Geometry check sheet. Reference: the model listing, model coordinates, mm. A direction names the side the tool comes from. Coordinates: 2 decimals unless noted, no trailing zeros. Write each loop counter-clockwise with the first axis right and the second up, starting at its lowest first coordinate (ties: lowest second). Pieces come first, ordered by that corner, then holes. Notation, with made-up numbers: M -19.75,67.5 L 36.25,67.5 A16 ccw 36.25,88.5 Z; hole C 71.25,-27 d3. An arc over 180 degrees is marked long. Write each question's results on one line, items separated by ' | '.
```python
from build123d import *

# Parameters (mm, degrees)
BOSS_EXTRUDE1_DEPTH = 38.1
SKETCH2_W           = 38.1
SKETCH2_H           = 22.225
BOSS_EXTRUDE2_DEPTH = 25.4
CUT_EXTRUDE1_DEPTH  = 25.4


with BuildPart() as part:
    # Sketch1 → Boss-Extrude1 (new body, symmetric)
    with BuildSketch(Plane(origin=(0, 0, 0), x_dir=(0, 0, -1), z_dir=(1, 0, 0))):
        Polygon((-10.0584, -30.4038), (8.9916, -30.4038), (8.9916, -52.6288), (34.3916, -52.6288), (34.3916, 14.0462), (8.9916, 14.0462), (8.9916, -8.1788), (-10.0584, -8.1788), align=None)
    extrude(amount=BOSS_EXTRUDE1_DEPTH, both=True)

    # Sketch2 → Boss-Extrude2 (add)
    with BuildSketch(Plane.XY.offset(10.0584)):
        with Locations((0, -19.2913)):
            Rectangle(SKETCH2_W, SKETCH2_H)
    extrude(amount=BOSS_EXTRUDE2_DEPTH)

    # Sketch3 → Cut-Extrude1 (cut)
    with BuildSketch(Plane.XY.offset(-8.9916)):
        Polygon((6.35, -1.8288), (25.4, 14.0462), (-25.4, 14.0462), (-6.35, -1.8288), (-6.35, -8.1788), (6.35, -8.1788), align=None)
    extrude(amount=-CUT_EXTRUDE1_DEPTH, mode=Mode.SUBTRACT)


solid = part.part
```
Q1. Scan lines: probe 1 along Y at (x, z) = (33, 4.5); probe 2 along X at (y, z) = (-27.5, 26); probe 3 along Z at (x, y) = (-20.5, -20.5). Record each from-to range of solid material in increasing order.
Geometry check:
probe 1: y = -30.4 to -8.18 | probe 2: x = -19.05 to 19.05 | probe 3: z = -34.39 to 10.06
Q2. Access from +Z, -Z, +X, -X, +Y, -Y to the whole of each face (thin tool, end or side, straight path). Record for faces 1 (the flat face through (-28, -19, 10.058)), 2 (the flat face through (1, -30.404, 9)), 3 (the flat face through (29, -19, 10.058)), 4 (the flat face through (-26, 1, -8.992)).
Geometry check:
face 1: +Z, -X, +Y, -Y | face 2: +Z, +X, -X, -Y | face 3: +Z, +X, +Y, -Y | face 4: +Z, +X, -X, +Y
Q3. Mould release check, pull along X, two halves, no side actions. Record for faces 5 (the flat face through (15.742, 5.998, -21.514)), 6 (the flat face through (-19.05, -19, 23)), 7 (the flat face through (-32, 14.046, -22)): pulls with the +X half, pulls with the -X half, needs draft (parallel to the pull), parting line crosses it, or undercut.
Geometry check:
face 5: undercut | face 6: pulls with the -X half | face 7: needs draft
Q4. Sectioned sample at C-C on z = -11.5. Record the cut outline in (x, y), and give its area (3 significant figures).
Geometry check:
outline: M -38.1,-52.63 L 38.1,-52.63 L 38.1,14.05 L 25.4,14.05 L 6.35,-1.83 L 6.35,-8.18 L -6.35,-8.18 L -6.35,-1.83 L -25.4,14.05 L -38.1,14.05 Z | area: 4,500 mm2
Q5. Sectioned sample at D-D on y = -26. Record the cut outline in (x, z), and give its area (3 significant figures).
Geometry check:
outline: M -38.1,-34.39 L 38.1,-34.39 L 38.1,10.06 L 19.05,10.06 L 19.05,35.46 L -19.05,35.46 L -19.05,10.06 L -38.1,10.06 Z | area: 4,350 mm2
Q6. Sectioned sample at A-A on x = 27. Record the cut outline in (y, z), and give its area (3 significant figures).
Geometry check:
outline: M -52.63,-34.39 L 14.05,-34.39 L 14.05,-8.99 L -8.18,-8.99 L -8.18,10.06 L -30.4,10.06 L -30.4,-8.99 L -52.63,-8.99 Z | area: 2,120 mm2
Q7. Sectioned sample at B-B on y = 3. Record the cut outline in (x, z).
Geometry check:
outline: M -38.1,-34.39 L -12.14,-34.39 L -12.14,-8.99 L -38.1,-8.99 Z; M 12.14,-34.39 L 38.1,-34.39 L 38.1,-8.99 L 12.14,-8.99 Z
Q8. Depth check by flat-ended pin: P1, Ø3, axis at x = -26, y = -38.5, coming from the +Z side; P2, Ø24.5, axis at y = -21, z = 19.5, coming from the +X side; P3, Ø5.5, axis at x = 33, y = -24, coming from the +Z side; P4, Ø4, axis at y = -4.5, z = 19.5, coming from the +X side. Enter the tip coordinate at first touch or a pass-through.
Geometry check:
P1: stops at z = -8.99 | P2: stops at x = 38.1 | P3: stops at z = 10.06 | P4: passes through
